The figure shows three views and two pictorial views of one solid part (mm, origin at its lowest corner). Answer the questions. Round coordinates to 2 decimals unless told otherwise and drop trailing zeros. Write each loop counter-clockwise with the first axis right and the second up, starting at its lowest first coordinate (ties: lowest second). Pieces come first, ordered by that corner, then holes. Notation, with made-up numbers: (57, 73) -> (63, 73) arc R25 cw to (63, 87) -> close; hole circle Ø10 at (2.25, -23.5). An arc over 180 degrees is marked (long way). One line per item, written item: value.
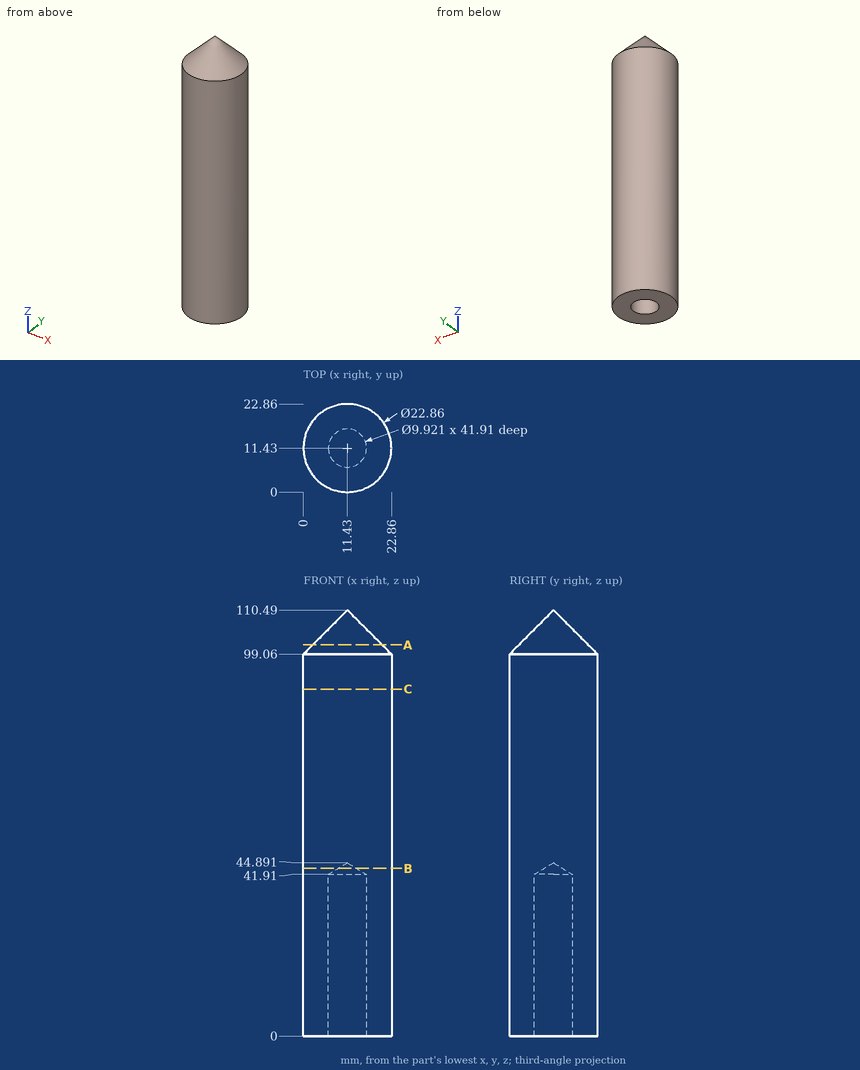
(1) Flat-ended cylindrical pins translate along their axes: pin 1 Ø1.5 at (x, z) = (4, 22) entering from +Y (1 decimal); pin 2 Ø6 at (x, y) = (20, 15.5) entering from -Z; pin 3 Ø1.5 at (x, z) = (17.5, 44) entering from -Y; pin 4 Ø12 at (y, z) = (5, 31) entering from -X. Find the tip coordinate at first contact, or state that the pin passes through.
Reported:
pin 1: stops at y = 20.7
pin 2: stops at z = 0
pin 3: stops at y = 1.31
pin 4: stops at x = 0.01
(2) Consider probe 1 along Y at (x, z) = (11.43, 29); probe 2 along X at (y, z) = (8.5, 9); probe 3 along Z at (x, y) = (7.5, 18.25). Determine where each line is inside the solid, lowest interval first.
Reported:
probe 1: y = 0 to 6.47, 16.39 to 22.86
probe 2: x = 0.38 to 7.43, 15.43 to 22.48
probe 3: z = 0 to 102.62
(3) Find section C-C on z = 90. Give the vertices of the cut face in (x, y).
Reported:
outline: circle Ø22.86 at (11.43, 11.43)
(4) Find section B-B on z = 43.5. Give the vertices of the cut face in (x, y) (1 decimal), plus the area to 3 significant figures.
Reported:
outline: circle Ø22.9 at (11.4, 11.4); hole circle Ø4.6 at (11.4, 11.4)
area: 394 mm2
(5) Find section A-A on z = 101.5. Give the vertices of the cut face in (x, y).
Reported:
outline: circle Ø17.98 at (11.43, 11.43)
